Geometry check sheet. Reference: the model listing, model coordinates, mm. Face numbers are marked on the shaded views. A direction names the side the tool comes from. Round coordinates to 2 decimals unless told otherwise and drop trailing zeros. Order: outer loops, then holes, each group sorted by start corner. A loop starts at its lowest first (then second) coordinate and runs counter-clockwise, first axis right, second up. Notation, with made-up numbers: (19, -19.5) -> (65, -19.5) arc R22 ccw to (65, -6.5) -> close; hole circle Ø6 at (54.5, 49). An arc over 180 degrees is marked (long way). Use a Markdown table: item, result. Add a question column.
Item 1: Sectioned sample at C-C, the plane y = 30. State how many separate pieces and enclosed holes the cut face has, and give its area (3 significant figures).
Item 2: Material ranges on probe 1 along Z at (x, y) = (0, 2); probe 2 along X at (y, z) = (38, 3); probe 3 along X at (y, z) = (33, -53.5), recorded low to high. Write a range as [from, to].
Item 3: Sectioned sample at A-A, the plane y = 44. Record the cut outline in (x, z), and give its area (3 significant figures).
Item 4: Mould release check, pull along X, two halves, no side actions. Record for the marked faces 5, 6 and 7: pulls with the +X half, pulls with the -X half, needs draft (parallel to the pull), parting line crosses it, or undercut.
Item 5: Set-up check for the marked faces 1, 2, 3 and 4: record each of +Z, -Z, +X, -X, +Y, -Y from which the full face is reachable in a straight line by a thin tool's end or side.
Item 6: Sectioned sample at B-B, the plane z = -36.5. Record the cut outline in (x, y).
Item 7: Gauge pin test, flat ends, axial feed: pin 1 Ø4 at (x, z) = (-44.5, -37.5) entering from -Y; pin 2 Ø5 at (x, z) = (2, 10) entering from +Y; pin 3 Ø4 at (x, y) = (-60, 27.5) entering from +Z; pin 4 Ø1.3 at (y, z) = (19.5, 54) entering from -X. Record the tip position at first contact, or that the pin passes through.
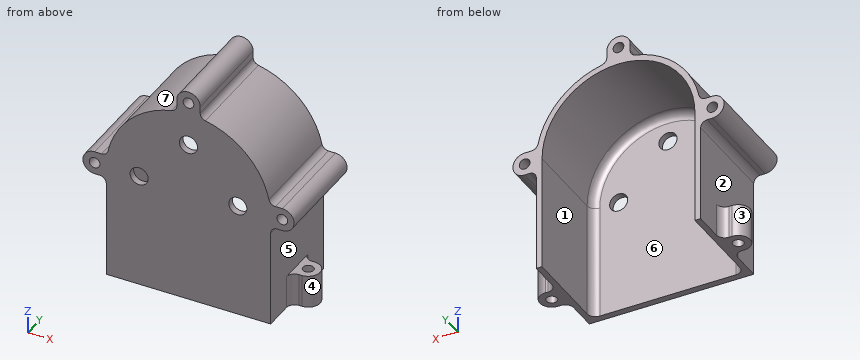
Autodesk Inventor part; units mm, degrees
ref_plane "YZ Plane" through (0, 0, 0) normal (1, 0, 0) x (0, 1, 0)
ref_plane "XZ Plane" through (0, 0, 0) normal (0, 1, 0) x (-1, 0, 0)
ref_plane "XY Plane" through (0, 0, 0) normal (0, 0, 1) x (1, 0, 0)
sketch "Sketch1" plane through (0, 0, 0) normal (0, 1, 0) x (-1, 0, 0)
  arc A0 (-10.2866, 48.9304) -> (-48.9304, 10.2866) centre (0, 0) ccw
  circle A1 centre (30, 0) radius 5.5
  circle A2 centre (0, 30) radius 5.5
  circle A3 centre (-30, 0) radius 5.5
  line L0 (50, -11.1096) -> (50, -70)
  line L1 (50, -70) -> (-50, -70)
  line L2 (-50, -70) -> (-50, -11.1096)
  line L3 (-46.5, 0) -> (-46.5, -70)
  line L4 (46.5, -70) -> (46.5, 0)
  arc A4 (46.5, 0) -> (-46.5, 0) centre (0, 0) ccw
  circle A5 centre (57.1096, 0) radius 3.25
  circle A6 centre (57.1096, 0) radius 7.1096
  line L5 (57.1096, -7.1096) -> (54, -7.1096)
  line L6 (57.1096, 7.1096) -> (52.8448, 7.1096)
  circle A7 centre (0, 57.1096) radius 7.1096
  circle A8 centre (0, 57.1096) radius 3.25
  circle A9 centre (-57.1096, 0) radius 7.1096
  circle A10 centre (-57.1096, 0) radius 3.25
  line L7 (-57.1096, -7.1096) -> (-54, -7.1096)
  line L8 (-57.1096, 7.1096) -> (-52.8448, 7.1096)
  line L9 (-7.1096, 57.1096) -> (-7.1096, 52.8448)
  line L10 (7.1096, 57.1096) -> (7.1096, 52.8448)
  arc A11 (48.9304, 10.2866) -> (52.8448, 7.1096) centre (52.8448, 11.1096) ccw
  arc A12 (-52.8448, 7.1096) -> (-48.9304, 10.2866) centre (-52.8448, 11.1096) ccw
  arc A13 (-10.2866, 48.9304) -> (-7.1096, 52.8448) centre (-11.1096, 52.8448) ccw
  arc A14 (54, -7.1096) -> (50, -11.1096) centre (54, -11.1096) ccw
  arc A15 (-50, -11.1096) -> (-54, -7.1096) centre (-54, -11.1096) ccw
  arc A16 (48.9304, 10.2866) -> (10.2866, 48.9304) centre (0, 0) ccw
  arc A17 (7.1096, 52.8448) -> (10.2866, 48.9304) centre (11.1096, 52.8448) ccw
  point P0 (50, 0)
  point P1 (-50, 0)
  point P2 (49.492, 7.1096)
  point P3 (-49.492, 7.1096)
  point P4 (-7.1096, 49.492)
  point P5 (7.1096, 49.492)
  dimension "d0" = 100
  dimension "d1" = 11
  dimension "d2" = 30
  dimension "d5" = 180
  dimension "d7" = 3.5
  dimension "d8" = 70
  dimension "d9" = 6.5
  dimension "d12" = 180
  dimension "d14" = 4
  dimension "d15" = 4
extrude "Extrusion1" add sketch "Sketch1" along normal blind 4 contours L3 A4 L4 L1
extrude "Extrusion2" add sketch "Sketch1" along normal blind 60 contours A13 L9 A7 L10 A17 A16 A11 L6 A6 L5 A14 L0 L1 L4 A4 L3 L2 A15 L7 A9 L8 A12 A0 | A7 | A9 | A6
ref_plane "Work Plane1" through (0, 0, -11.1096) normal (1, 0, 0) x (0, 0, -1)
sketch "Sketch2" plane through (50, 0, -70) normal (0, 0, -1) x (-1, 0, 0)
  circle A0 centre (-6.7309, 30) radius 3.25
  arc A1 (-6.7309, 37.25) -> (-6.7309, 22.75) centre (-6.7309, 30) ccw
  line L0 (-6.7309, 37.25) -> (0, 37.25)
  line L1 (0, 0) -> (0, 60)
  line L2 (-6.7309, 22.75) -> (0, 22.75)
  line L3 (0, 37.25) -> (0, 22.75)
  line L4 (0, 60) -> (3.5, 60)
  point P0 (50, 0)
  dimension "d20" = 6.5
  dimension "d21" = 4
  dimension "d22" = 30
  dimension "d23" = 60
extrude "Extrusion3" add sketch "Sketch2" against normal blind 20
fillet "Fillet1" radius 5 2 edges at (50, 37.25, -60) (50, 22.75, -60)
mirror "Mirror1" about plane through (0, 0, -11.1096) normal (1, 0, 0) of "Extrusion3"
fillet "Fillet2" radius 5 2 edges at (-50, 37.25, -60) (-50, 22.75, -60)
fillet "Fillet3" radius 5 3 edges at (0, 4, 46.5) (46.5, 4, -35) (-46.5, 4, -35)
equation "\"d22\" = 0.5 * d23"
properties part number "Fej"
Found:
| question | item | result |
|---|---|---|
| 1 | separate pieces | 3 |
| 1 | enclosed holes | 3 |
| 1 | area | 1,780 mm2 |
| 2 | probe 1 | z = [-70, 24.5], [35.5, 53.86], [60.36, 64.22] |
| 2 | probe 2 | x = [-63.56, -58.36], [-55.86, -46.4], [46.4, 55.86], [58.36, 63.56] |
| 2 | probe 3 | x = [-63.33, -57.98], [-55.48, -46.5], [46.5, 55.48], [57.98, 63.33] |
| 3 | outline | (-57.11, -7.11) -> (-54, -7.11) arc R4 cw to (-50, -11.11) -> (-50, -70) -> (-46.5, -70) -> (-46.5, 0) arc R46.5 cw to (46.5, 0) -> (46.5, -70) -> (50, -70) -> (50, -11.11) arc R4 cw to (54, -7.11) -> (57.11, -7.11) arc R7.11 ccw to (57.11, 7.11) -> (52.84, 7.11) arc R4 cw to (48.93, 10.29) arc R50 ccw to (10.29, 48.93) arc R4 cw to (7.11, 52.84) -> (7.11, 57.11) arc R7.11 ccw to (-7.11, 57.11) -> (-7.11, 52.84) arc R4 cw to (-10.29, 48.93) arc R50 ccw to (-48.93, 10.29) arc R4 cw to (-52.84, 7.11) -> (-57.11, 7.11) arc R7.11 ccw to start; hole circle Ø6.5 at (-57.11, 0); hole circle Ø6.5 at (0, 57.11); hole circle Ø6.5 at (57.11, 0) |
| 3 | area | 1,480 mm2 |
| 4 | face 5 | pulls with the +X half |
| 4 | face 6 | undercut |
| 4 | face 7 | pulls with the -X half |
| 5 | face 1 | -Z, +Y |
| 5 | face 2 | -X |
| 5 | face 3 | -Z, -X |
| 5 | face 4 | -Z, +X |
| 6 | outline | (-50, 0) -> (50, 0) -> (50, 60) -> (46.5, 60) -> (46.5, 9) arc R5 cw to (41.5, 4) -> (-41.5, 4) arc R5 cw to (-46.5, 9) -> (-46.5, 60) -> (-50, 60) -> close |
| 7 | pin 1 | stops at y = 0 |
| 7 | pin 2 | stops at y = 4 |
| 7 | pin 3 | stops at z = 7.05 |
| 7 | pin 4 | stops at x = -7.11 |
